Drawing for the job (mm, zero at the part's lowest x, y, z). Round coordinates to 2 decimals unless told otherwise and drop trailing zeros. Loops run counter-clockwise (first coordinate to the right, second up) from the corner with the lowest first, then second, coordinate; pieces in that order, holes last. Notation, with made-up numbers: (-24, -35) -> (12, -35) arc R33 ccw to (12, -6) -> close; hole circle Ø8 at (-20, 75.25). An arc over 180 degrees is marked (long way). Put each result on its own line as item: value. Start each with the question number.
Item 1: Cut at B-B, the plane z = 52.5. List the corners of the cut face in (x, y), plus the area to 3 significant figures.
Item 2: Flat gauge pin, fed straight in: pin 1 Ø2.5 at (x, z) = (61.5, 52.5) entering from +Y. Where does the tip first touch, or does it go through?
Item 3: Drill centre lines: probe 1 along X at (y, z) = (3, 3.5); probe 2 along X at (y, z) = (11.75, 4.5). Where is each one in solid material? Low to high. Write a range as [from, to].
Item 4: Cut at A-A, the plane x = 3.5. List the corners of the cut face in (y, z).
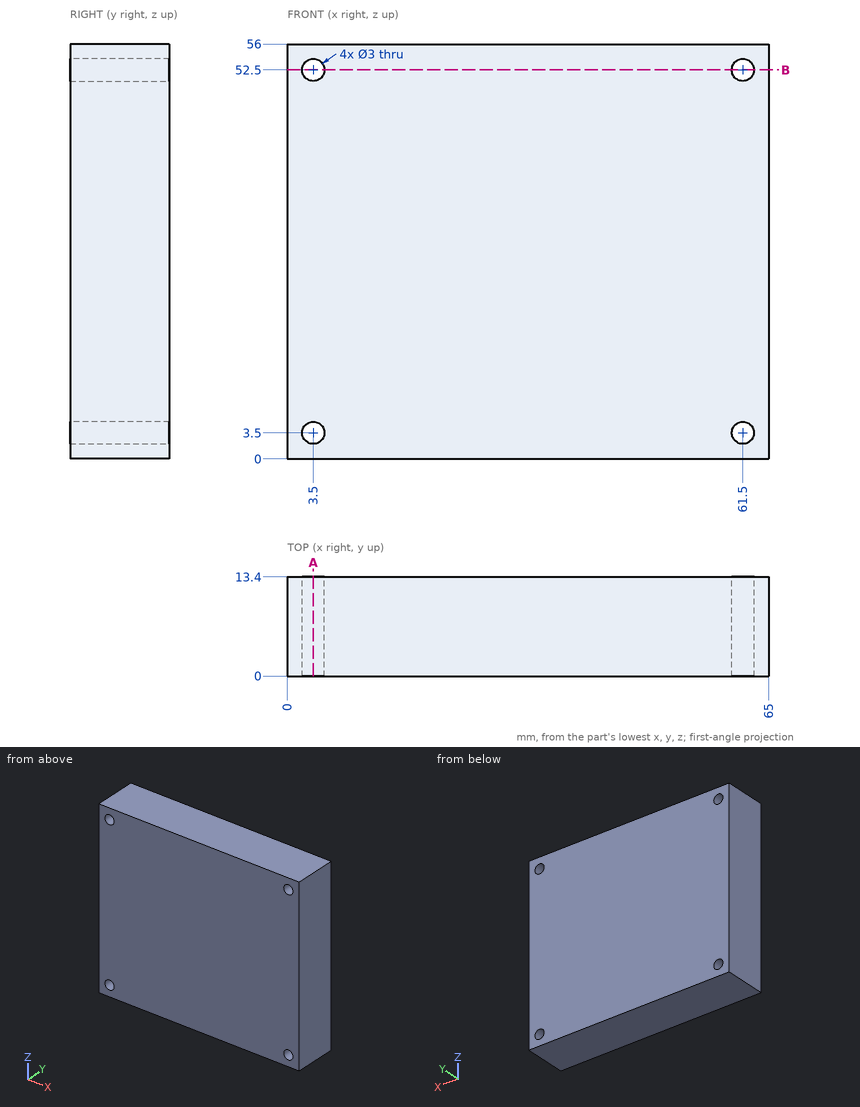
Reply:
1. outline: (0, 0) -> (2, 0) -> (2, 13.4) -> (0, 13.4) -> close; (5, 0) -> (60, 0) -> (60, 13.4) -> (5, 13.4) -> close; (63, 0) -> (65, 0) -> (65, 13.4) -> (63, 13.4) -> close
1. area: 791 mm^2
2. pin 1: passes through
3. probe 1: x = [0, 2], [5, 60], [63, 65]
3. probe 2: x = [0, 2.38], [4.62, 60.38], [62.62, 65]
4. outline: (0, 0) -> (13.4, 0) -> (13.4, 2) -> (0, 2) -> close; (0, 5) -> (13.4, 5) -> (13.4, 51) -> (0, 51) -> close; (0, 54) -> (13.4, 54) -> (13.4, 56) -> (0, 56) -> close
